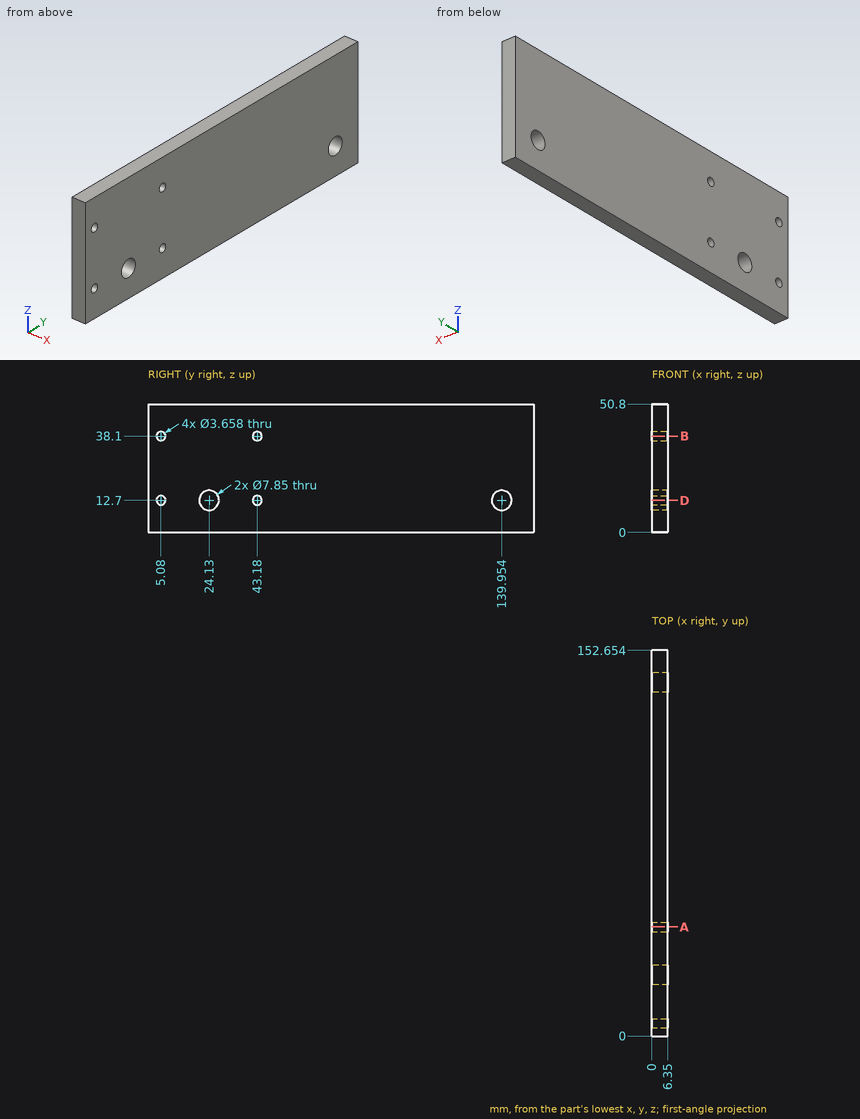
Geometry: see drawing. Coordinates: mm, zero at the bounding-box minimum. Round coordinates to 2 decimals unless told otherwise and drop trailing zeros. Loops run counter-clockwise (first coordinate to the right, second up) from the corner with the lowest first, then second, coordinate; pieces in that order, holes last. Notation, with made-up numbers: (79, 1.25) - (119, 1.25) arc R16 cw to (119, 32.25) - close; hole circle Ø3 at (76.5, 30). An arc over 180 degrees is marked (long way). Write item = value, one per line. Start each with the question number.
(1) Pin query (flat end, axial travel): pin 1 (1 mm diameter, centred on x = 2, z = 41, fed in from -Y); pin 2 (7 mm diameter, centred on y = 139.954, z = 12.7, fed in from +X). Return the tip coordinate at first contact, or that it passes through.
(2) Section query A-A, the plane y = 43.18. Output: boundary loops of the cut face in (x, z), plus the area to 3 significant figures.
(3) Ray query, line 1 along Y through (x, z) = (4, 12.7) (1 decimal); line 2 along Y through (x, z) = (4, 38.1); line 3 along Y through (x, z) = (2.25, 37) (1 decimal). Return the intervals inside material, ascending. Write a range as from..to.
(4) Section query D-D, the plane z = 12.7. State how many separate pieces and enclosed holes the cut face has, plus the area to 3 significant figures.
(5) Section query B-B, the plane z = 38.1. Output: boundary loops of the cut face in (x, y).
Conclusion:
q1.pin_1 = 0
q1.pin_2 = through
q2.outline = (0, 0) - (6.35, 0) - (6.35, 10.87) - (0, 10.87) - close; (0, 14.53) - (6.35, 14.53) - (6.35, 36.27) - (0, 36.27) - close; (0, 39.93) - (6.35, 39.93) - (6.35, 50.8) - (0, 50.8) - close
q2.area = 276 mm2
q3.line_1 = 0..3.3, 6.9..20.2, 28.1..41.4, 45..136, 143.9..152.7
q3.line_2 = 0..3.25, 6.91..41.35, 45.01..152.65
q3.line_3 = 0..3.6, 6.5..41.7, 44.6..152.7
q4.separate_pieces = 5
q4.enclosed_holes = 0
q4.area = 823 mm2
q5.outline = (0, 0) - (6.35, 0) - (6.35, 3.25) - (0, 3.25) - close; (0, 6.91) - (6.35, 6.91) - (6.35, 41.35) - (0, 41.35) - close; (0, 45.01) - (6.35, 45.01) - (6.35, 152.65) - (0, 152.65) - close
